```python
from build123d import *

# Parameters (mm, degrees)
SKETCH1_W           = 52
SKETCH1_H           = 33.5
COVER_PLATE_DEPTH   = 3
SKETCH2_W           = 31
SKETCH2_H           = 17
LOCATING_PLUG_DEPTH = 2.41
SKETCH3_R           = 1.7
SCREW_HOLES_DEPTH   = 5


with BuildPart() as part:
    # Sketch1 → Cover Plate (new body)
    with BuildSketch(Plane(origin=(-75.4, 0, 0), x_dir=(0, 0, -1), z_dir=(1, 0, 0))):
        with Locations((-64, -10.25)):
            Rectangle(SKETCH1_W, SKETCH1_H)
    extrude(amount=COVER_PLATE_DEPTH)

    # Sketch2 → Locating Plug (add)
    with BuildSketch(Plane(origin=(-72.41, 0, 0), x_dir=(0, 0, -1), z_dir=(1, 0, 0))):
        with Locations((-64, -9)):
            Rectangle(SKETCH2_W, SKETCH2_H)
    extrude(amount=LOCATING_PLUG_DEPTH)

    # Sketch3 → Screw Holes (cut)
    with BuildSketch(Plane(origin=(-76.4, 0, 0), x_dir=(0, 0, -1), z_dir=(1, 0, 0))):
        with Locations((-86, -23)):
            Circle(SKETCH3_R)
        with Locations((-86, 3)):
            Circle(SKETCH3_R)
        with Locations((-42, -23)):
            Circle(SKETCH3_R)
        with Locations((-42, 3)):
            Circle(SKETCH3_R)
    extrude(amount=SCREW_HOLES_DEPTH, mode=Mode.SUBTRACT)


solid = part.part
```
Geometry check sheet. Reference: the model listing, model coordinates, mm. A direction names the side the tool comes from. Coordinates: 2 decimals unless noted, no trailing zeros. Order: outer loops, then holes, each group sorted by start corner. A loop starts at its lowest first (then second) coordinate and runs counter-clockwise, first axis right, second up. Notation, with made-up numbers: M 31,35 L 54,35 A15 ccw 54,53 Z; hole C 7,52.5 d7. An arc over 180 degrees is marked long. One line per question, with ' | ' between items. Start each with the question number.
Item 1: Draft check along Z on faces 1 (the cylindrical face through (-73.92, -21.85, 43.25)), 2 (the flat face through (-71, -9, 48.5)), 3 (the flat face through (-70, -9, 64)). Enter one of: pulls with the +Z half, pulls with the -Z half, needs draft (parallel to the pull), parting line crosses it, or undercut.
Item 2: Cross-section at B-B on z = 86. Enter the section's corners in (x, y).
Item 3: Cross-section at A-A on y = 3. Enter the section's corners in (x, z), then the cut area to 3 significant figures.
Item 4: Gauge pin test, flat ends, axial feed: pin 1 (3 mm diameter, centred on y = -23, z = 42, fed in from -X); pin 2 (5.5 mm diameter, centred on y = 3, z = 86, fed in from +X); pin 3 (1.9 mm diameter, centred on x = -71, y = -9, fed in from +Z); pin 4 (0.7 mm diameter, centred on x = -71, z = 58, fed in from -Y). Record the tip position at first contact, or that the pin passes through.
Item 5: Cross-section at D-D on x = -73.5. Enter the section's corners in (y, z).
Item 6: Cross-section at C-C on z = 69.5. Enter the section's corners in (x, y), then the cut area to 3 significant figures.
Item 7: Material ranges on L1, parallel to Z at x = -73.2, y = -23; L2, parallel to Y at x = -73.5, z = 86; L3, parallel to Z at x = -74.75, y = -22, recorded low to high. Write a range as [from, to].
Item 8: Set-up check for faces 4 (the flat face through (-71, -9, 79.5)), 5 (the flat face through (-71, -0.5, 64)), 6 (the flat face through (-71, -17.5, 64)): record each of +Z, -Z, +X, -X, +Y, -Y from which the full face is reachable in a straight line by a thin tool's end or side.
Findings:
1) face 1: undercut | face 2: pulls with the -Z half | face 3: needs draft
2) outline: M -75.4,-27 L -72.4,-27 L -72.4,-24.7 L -75.4,-24.7 Z; M -75.4,-21.3 L -72.4,-21.3 L -72.4,1.3 L -75.4,1.3 Z; M -75.4,4.7 L -72.4,4.7 L -72.4,6.5 L -75.4,6.5 Z
3) outline: M -75.4,38 L -72.4,38 L -72.4,40.3 L -75.4,40.3 Z; M -75.4,43.7 L -72.4,43.7 L -72.4,84.3 L -75.4,84.3 Z; M -75.4,87.7 L -72.4,87.7 L -72.4,90 L -75.4,90 Z | area: 136 mm²
4) pin 1: passes through | pin 2: stops at x = -72.4 | pin 3: stops at z = 79.5 | pin 4: stops at y = -17.5
5) outline: M -27,38 L 6.5,38 L 6.5,90 L -27,90 Z; hole C -23,42 d3.4; hole C -23,86 d3.4; hole C 3,42 d3.4; hole C 3,86 d3.4
6) outline: M -75.4,-27 L -72.4,-27 L -72.4,-17.5 L -70,-17.5 L -70,-0.5 L -72.4,-0.5 L -72.4,6.5 L -75.4,6.5 Z | area: 141 mm²
7) L1: z = [38, 40.3], [43.7, 84.3], [87.7, 90] | L2: y = [-27, -24.7], [-21.3, 1.3], [4.7, 6.5] | L3: z = [38, 40.63], [43.37, 84.63], [87.37, 90]
8) face 4: +Z, +X, +Y, -Y | face 5: +Z, -Z, +X, +Y | face 6: +Z, -Z, +X, -Y
